Here's how the part is built. I have some questions about the finished solid (model axes, mm). A direction names the side the tool comes from. Round coordinates to 2 decimals unless told otherwise and drop trailing zeros. Order: outer loops, then holes, each group sorted by start corner. A loop starts at its lowest first (then second) coordinate and runs counter-clockwise, first axis right, second up.
```python
from build123d import *

# Parameters (mm, degrees)
F3_SIZE  = 1.27
F4_SIZE  = 0.254
F5_W     = 4.7752
F5_H     = 2.54
F6_DEPTH = 193.675
F8_DEPTH = 1.1938


with BuildPart() as f2:
    # F0 (on Front) → F2 (revolve)
    with BuildSketch(Plane.XZ):
        Polygon((0, 12.7), (0, 0), (203.2, 0), (203.2, 6.35), (145.135334, 11.43), (15.875, 11.43), (15.875, 10.16), (9.525, 10.16), (9.525, 12.7), align=None)
    revolve(axis=Axis((47.973725, 0, 0), (1, 0, 0)))

    # F3
    f3_edges = [f2.edges().sort_by_distance(p)[0] for p in [
        (0, 0, -12.7),
    ]]
    chamfer(f3_edges, length=F3_SIZE)

    # F4
    f4_edges = [f2.edges().sort_by_distance(p)[0] for p in [
        (203.2, 0, -6.35),
    ]]
    chamfer(f4_edges, length=F4_SIZE)

    # F5 (on face) → F6 (cut, through all)
    with BuildSketch(Plane.YZ.offset(203.2)):
        with Locations((0, 10.16)):
            Rectangle(F5_W, F5_H)
        with Locations((0, -10.16)):
            Rectangle(F5_W, F5_H)
    extrude(amount=-F6_DEPTH, mode=Mode.SUBTRACT)

    # F7 (on Top) → F8 (cut, symmetric)
    with BuildSketch(Plane.XY):
        Polygon((28.575, 11.637617), (180.941923, 8.462617), (180.941923, 11.637617), align=None)
        Polygon((180.941923, -8.462617), (28.575, -11.637617), (180.941923, -11.637617), align=None)
    extrude(amount=F8_DEPTH, both=True, mode=Mode.SUBTRACT)


solid = f2.part
```
1. I'm going to push flat-ended pins straight in: P1, Ø2.5, axis at x = 120.5, y = -9.5, coming from the -Z side; P2, Ø4, axis at x = 98.5, y = -1, coming from the -Z side; P3, Ø7.5, axis at y = 4.5, z = -6, coming from the +X side; P4, Ø1.8, axis at x = 105, z = -10, coming from the -Y side. Where does each tip first touch, or does it pass through?
Evaluation:
P1: stops at z = -7.91
P2: stops at z = -11.18
P3: stops at x = 203.2
P4: stops at y = -6.92
2. On a 3-axis mill with a long thin cutter (end or side, diameter ignored), from which of +Z, -Z, +X, -X, +Y, -Y can I reach the whole of each face in a straight line? I mean faces 1 (the cylindrical face through (12.66, -10.16, 0.19)), 2 (the cylindrical face through (79.6, -10.845, 3.61)), 3 (the flat face through (9.525, -1.9, -9.3)), 4 (the flat face through (93, 0, -8.89)), 5 (the flat face through (15.875, 11, 0)). Say none if no direction works.
Evaluation:
face 1: -Y
face 2: +X, -Y
face 3: none
face 4: -Z, +X
face 5: +Y
3. If we section it at B-B, the plane x = 31.5: Write out the boundary of the cut face in (y, z), and give its area (3 significant figures).
Evaluation:
outline: (-2.39, -11.18) - (-2.39, -8.89) - (2.39, -8.89) - (2.39, -11.18) arc R11.43 ccw to (2.39, 11.18) - (2.39, 8.89) - (-2.39, 8.89) - (-2.39, 11.18) arc R11.43 ccw to start
area: 387 mm2
4. If we section it at A-A, the plane y = 0: Write out the boundary of the cut face in (x, z) (3 decimals), and give its area (3 significant figures).
Evaluation:
outline: (0, -11.43) - (1.27, -12.7) - (9.525, -12.7) - (9.525, -8.89) - (174.168, -8.89) - (202.947, -6.372) - (203.2, -6.096) - (203.2, 6.096) - (202.947, 6.372) - (174.168, 8.89) - (9.525, 8.89) - (9.525, 12.7) - (1.27, 12.7) - (0, 11.43) - close
area: 3,610 mm2
5. If we section it at C-C, the plane x = 73: Write out the boundary of the cut face in (y, z).
Evaluation:
outline: (-11.37, -1.19) arc R11.43 ccw to (-2.39, -11.18) - (-2.39, -8.89) - (2.39, -8.89) - (2.39, -11.18) arc R11.43 ccw to (11.37, -1.19) - (10.71, -1.19) - (10.71, 1.19) - (11.37, 1.19) arc R11.43 ccw to (2.39, 11.18) - (2.39, 8.89) - (-2.39, 8.89) - (-2.39, 11.18) arc R11.43 ccw to (-11.37, 1.19) - (-10.71, 1.19) - (-10.71, -1.19) - close
6. If we section it at D-D, the plane x = 139.5: Write out the boundary of the cut face in (y, z), and give its area (3 significant figures).
Evaluation:
outline: (-11.37, -1.19) arc R11.43 ccw to (-2.39, -11.18) - (-2.39, -8.89) - (2.39, -8.89) - (2.39, -11.18) arc R11.43 ccw to (11.37, -1.19) - (9.33, -1.19) - (9.33, 1.19) - (11.37, 1.19) arc R11.43 ccw to (2.39, 11.18) - (2.39, 8.89) - (-2.39, 8.89) - (-2.39, 11.18) arc R11.43 ccw to (-11.37, 1.19) - (-9.33, 1.19) - (-9.33, -1.19) - close
area: 377 mm2
7. I need wall thicknesses on probe 1 along Y at (x, z) = (50, -9.5); probe 2 along Z at (x, y) = (126, 10.5); probe 3 along Y at (x, z) = (124, -10). Which ranges of each line are inside material? Lowest first, please.
Evaluation:
probe 1: y = -6.36 to -2.39, 2.39 to 6.36
probe 2: z = -4.52 to -1.19, 1.19 to 4.52
probe 3: y = -5.54 to -2.39, 2.39 to 5.54
